The model under review builds one solid part; all positions refer to its coordinate system, in mm. A direction names the side the tool comes from. Round coordinates to 2 decimals unless told otherwise and drop trailing zeros. Loops run counter-clockwise (first coordinate to the right, second up) from the corner with the lowest first, then second, coordinate; pieces in that order, holes last. Notation, with made-up numbers: (48, 64.5) - (68, 64.5) arc R28 ccw to (68, 93.5) - close; hole circle Ø10 at (72.5, 45). An arc over 180 degrees is marked (long way). Answer as CSV lines item,"result".
from build123d import *

# Parameters (mm, degrees)
BOSS_EXTRUDE1_DEPTH = 22.7
SKETCH2_R           = 1.25
CUT_EXTRUDE1_DEPTH  = 3.5


with BuildPart() as part:
    # Sketch1 → Boss-Extrude1 (new, symmetric)
    with BuildSketch(Plane.XY):
        Polygon((-13.5, 2.506896552), (-6, 2.506896552), (-6, 8), (6, 8), (6, 2.506896552), (13.5, 2.506896552), (13.5, 12.506896552), (-13.5, 12.506896552), align=None)
    extrude(amount=BOSS_EXTRUDE1_DEPTH, both=True)

    # Sketch2 → Cut-Extrude1 (cut)
    with BuildSketch(Plane(origin=(0, 12.506896552, 0), x_dir=(1, 0, 0), z_dir=(0, 1, 0))):
        with Locations(Location((-10, 10, 0), (0, 0, 180))):
            Circle(SKETCH2_R)
        with Locations(Location((10, 10, 0), (0, 0, 180))):
            Circle(SKETCH2_R)
        with Locations(Location((-10, -10, 0), (0, 0, 180))):
            Circle(SKETCH2_R)
        with Locations(Location((10, -10, 0), (0, 0, 180))):
            Circle(SKETCH2_R)
    extrude(amount=-CUT_EXTRUDE1_DEPTH, mode=Mode.SUBTRACT)


solid = part.part
1. Take a section at B-B (z = 14). State the section outline as (x, y) points, plus the area to 3 significant figures.
Numbers:
outline,"(-13.5, 2.51) - (-6, 2.51) - (-6, 8) - (6, 8) - (6, 2.51) - (13.5, 2.51) - (13.5, 12.51) - (-13.5, 12.51) - close"
area,"204 mm²"
2. Take a section at D-D (z = -10). State the section outline as (x, y) points, plus the area to 3 significant figures.
Numbers:
outline,"(-13.5, 2.51) - (-6, 2.51) - (-6, 8) - (6, 8) - (6, 2.51) - (13.5, 2.51) - (13.5, 12.51) - (11.25, 12.51) - (11.25, 9.01) - (8.75, 9.01) - (8.75, 12.51) - (-8.75, 12.51) - (-8.75, 9.01) - (-11.25, 9.01) - (-11.25, 12.51) - (-13.5, 12.51) - close"
area,"187 mm²"
3. Take a section at C-C (x = 10). State the section outline as (y, z) points, plus the area to 4 significant figures.
Numbers:
outline,"(2.51, -22.7) - (12.51, -22.7) - (12.51, -11.25) - (9.01, -11.25) - (9.01, -8.75) - (12.51, -8.75) - (12.51, 8.75) - (9.01, 8.75) - (9.01, 11.25) - (12.51, 11.25) - (12.51, 22.7) - (2.51, 22.7) - close"
area,"436.5 mm²"
4. Tool access review of faces 4 (the face through (-6, 5, 0)), 5 (the face through (-10, 9.007, 10)), 6 (the face through (0, 9, -22.7)): name each direction out of +Z, -Z, +X, -X, +Y, -Y from which nothing blocks a thin tool from reaching the whole face with its end or side.
Numbers:
face 4,"+Z, -Z, -Y"
face 5,"+Y"
face 6,"-Z, +X, -X, +Y, -Y"
5. Take a section at A-A (y = 6.5). State the section outline as (x, z) points, plus the area to 3 significant figures.
Numbers:
outline,"(-13.5, -22.7) - (-6, -22.7) - (-6, 22.7) - (-13.5, 22.7) - close; (6, -22.7) - (13.5, -22.7) - (13.5, 22.7) - (6, 22.7) - close"
area,"681 mm²"
6. Clearance check with a flat-ended pin moving along its axis: pin 1 (1.5 mm diameter, centred on x = -10, z = 10, fed in from +Y). State where the tip first meets the part, or that it passes through.
Numbers:
pin 1,"stops at y = 9.01"
7. Draft analysis for pull direction X (two halves, no side actions). For faces 1 (the face through (13.5, 7, 0)), 2 (the face through (6, 5, 0)), 3 (the face through (10, 2.507, 0)), state which applies: +X half, -X half, draft (parallel to the pull), parting line (faces both ways), or undercut.
Numbers:
face 1,"+X half"
face 2,"undercut"
face 3,"draft"
8. Wall thickness on probe 1 along Z at (x, y) = (-10, 11.55); probe 2 along X at (y, z) = (7.75, -2); probe 3 along Y at (x, z) = (-2.25, -9.5): over which ranges is each line inside the solid? List them lowest first.
Numbers:
probe 1,"z = -22.7 to -11.25, -8.75 to 8.75, 11.25 to 22.7"
probe 2,"x = -13.5 to -6, 6 to 13.5"
probe 3,"y = 8 to 12.51"
